Answer from the drawing. Dimensions are ordinates in mm from the lowest x, y and z of the part. A direction names the side the tool comes from. Coordinates: 2 decimals unless noted, no trailing zeros. Order: outer loops, then holes, each group sorted by start corner. A loop starts at its lowest first (then second) coordinate and runs counter-clockwise, first axis right, second up. Notation, with made-up numbers: (41, -13) - (56, -13) arc R20 cw to (56, 25) - close; hole circle Ø7 at (10.5, 26.25). An arc over 180 degrees is marked (long way). Answer as a JSON object with one key per item and string values. Group by question number.
1) Section A-A (z = 11) is taken. Give the vertices of the cut face in (x, y).
2) The mould has two halves that part along Y. Classify the marked faces 4, 5 and 6: released by +Y, released by -Y, zero draft, split by the parting line, or undercut.
3) Each of these flat-tipped pins is pushed along its axis until it touches: P1, Ø1.2, axis at x = 10.5, z = 4, coming from the -Y side; P2, Ø4, axis at x = 17.5, y = 3.5, coming from the +Z side; P3, Ø0.6, axis at x = 16, z = 3, coming from the +Y side; P4, Ø12, axis at x = 10.5, y = 7.5, coming from the -Z side. Where does it stop, or does it pass through?
4) A tool of negligible diameter and unlimited length cuts with its end or side. For the marked faces 1, 2 and 3, from which of +Z, -Z, +X, -X, +Y, -Y can it reach the whole face along a straight path? Write none if from no direction.
5) Section B-B (z = 25.25) is taken. Give the vertices of the cut face in (x, y).
6) Find the intervals of material crossed by line 1 along X through (y, z) = (9, 5); line 2 along Z through (x, y) = (9.25, 17.75); line 3 along Z through (x, y) = (17.25, 11.5), in increasing order.
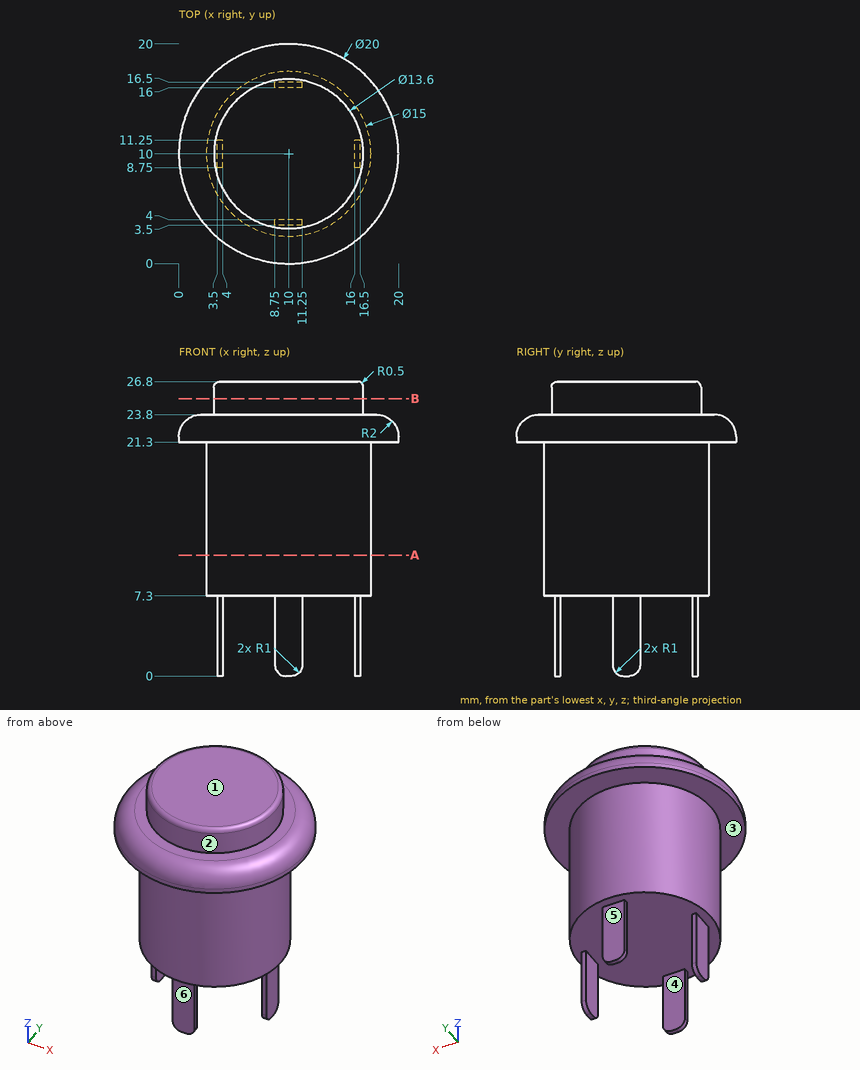
Report:
{
 "1": {"outline": "circle Ø15 at (10, 10)"},
 "2": {"face 4": "undercut", "face 5": "released by +Y", "face 6": "released by -Y"},
 "3": {"P1": "stops at y = 3.5", "P2": "stops at z = 23.8", "P3": "stops at y = 11.25", "P4": "stops at z = 0"},
 "4": {"face 1": "+Z, +X, -X, +Y, -Y", "face 2": "+Z", "face 3": "-Z"},
 "5": {"outline": "circle Ø13.6 at (10, 10)"},
 "6": {"line 1": "x = 3.5 to 4, 16 to 16.5", "line 2": "z = 21.3 to 23.8", "line 3": "z = 7.3 to 23.8"}
}
